Verification items for the finished model (mm, model axes). A direction names the side the tool comes from. Give positions to 0.01 mm unless a question says otherwise; leave off trailing zeros. Order: outer loops, then holes, each group sorted by start corner. A loop starts at its lowest first (then second) coordinate and runs counter-clockwise, first axis right, second up. Notation, with made-up numbers: (67.25, 17.25) - (99.25, 17.25) arc R27 ccw to (99.25, 46.25) - close; hole circle Ø2 at (2.25, 55). An arc over 180 degrees is marked (long way). Answer as a JSON object with one key per item and string values. Group by question number.
(1) Thickness scan on line 1 (Y direction, x = -239, z = 370); line 2 (Z direction, x = 136, y = -24). Record the ranges inside material, lowest first.
(2) Section check C-C (x = 239.5). Record the boundary of the cut face in (y, z), then the cut area to 3 significant figures.
(3) Mould release check, pull along Y, two halves, no side actions. Record for faces 4 (the face through (275.5, -4, 425)), 5 (the face through (-249, 223.3, 197)), 6 (the face through (-4, -275.5, 425)), 7 (the face through (-249, -223.3, 197)): +Y half, -Y half, draft (parallel to the pull), parting line (faces both ways), or undercut.
(4) Section check B-B (y = -133.5). Record the boundary of the cut face in (x, z).
(5) Depth check by flat-ended pin: pin 1 Ø13.5 at (y, z) = (240.5, 221) entering from -X; pin 2 Ø1 at (x, y) = (-216, 19.5) entering from -Z; pin 3 Ø23 at (y, z) = (-257, 281) entering from +X. Enter the tip coordinate at first touch or a pass-through.
(6) Access from +Z, -Z, +X, -X, +Y, -Y to the whole of each face (thin tool, end or side, straight path). Record for faces 1 (the face through (274, -249, 197)), 2 (the face through (-274, 248, 197)), 3 (the face through (248, -274, 197)).
(7) Section check A-A (z = 156). Count the separate pieces of the cut face and the enclosed holes in it, then the cut area to 3 significant figures.
```python
from build123d import *

# Parameters (mm, degrees)
F1_W     = 551
F1_H     = 551
F1_W_2   = 50.7
F1_H_2   = 50.7
F2_DEPTH = 50.1
F4_DEPTH = 400
F5_R     = 2.5
F6_R     = 1


with BuildPart() as f2:
    # F1 (on Top) → F2 (new body)
    with BuildSketch(Plane.XY):
        Rectangle(F1_W, F1_H)
        with Locations((-248.65, -248.65)):
            Rectangle(F1_W_2, F1_H_2, mode=Mode.SUBTRACT)
        with Locations((248.65, -248.65)):
            Rectangle(F1_W_2, F1_H_2, mode=Mode.SUBTRACT)
        with Locations((-248.65, 248.65)):
            Rectangle(F1_W_2, F1_H_2, mode=Mode.SUBTRACT)
        with Locations((248.65, 248.65)):
            Rectangle(F1_W_2, F1_H_2, mode=Mode.SUBTRACT)
        with Locations((-248.65, 248.65)):
            Rectangle(F1_W_2, F1_H_2)
        with Locations((248.65, 248.65)):
            Rectangle(F1_W_2, F1_H_2)
        with Locations((-248.65, -248.65)):
            Rectangle(F1_W_2, F1_H_2)
        with Locations((248.65, -248.65)):
            Rectangle(F1_W_2, F1_H_2)
    extrude(amount=-F2_DEPTH)


with BuildPart() as f2_1:
    # F3: moved
    add(f2.part.moved(Location((0, 0, 450))))

    # F1 (on Top) → F4 (join)
    with BuildSketch(Plane.XY):
        with Locations((-248.65, 248.65)):
            Rectangle(F1_W_2, F1_H_2)
        with Locations((248.65, -248.65)):
            Rectangle(F1_W_2, F1_H_2)
        with Locations((-248.65, -248.65)):
            Rectangle(F1_W_2, F1_H_2)
        with Locations((248.65, 248.65)):
            Rectangle(F1_W_2, F1_H_2)
    extrude(amount=F4_DEPTH)

    # F5
    f5_edges = [f2_1.edges().sort_by_distance(p)[0] for p in [
        (-274, -274, 199.95),
        (-274, 223.3, 199.95),
        (223.3, 223.3, 199.95),
        (223.3, -274, 199.95),
        (-223.3, -274, 199.95),
        (-223.3, 223.3, 199.95),
        (274, -274, 199.95),
        (274, 223.3, 199.95),
        (-223.3, -223.3, 199.95),
        (274, -223.3, 199.95),
        (-223.3, 274, 199.95),
        (274, 274, 199.95),
        (223.3, -223.3, 199.95),
        (-274, -223.3, 199.95),
        (223.3, 274, 199.95),
        (-274, 274, 199.95),
    ]]
    fillet(f5_edges, radius=F5_R)

    # F6
    f6_edges = [f2_1.edges().sort_by_distance(p)[0] for p in [
        (0, -275.5, 450),
        (275.5, 0, 450),
        (-275.5, 0, 450),
        (0, 275.5, 450),
        (275.5, -275.5, 424.95),
        (-275.5, -275.5, 424.95),
        (275.5, 275.5, 424.95),
        (-275.5, 275.5, 424.95),
    ]]
    fillet(f6_edges, radius=F6_R)


solid = f2_1.part
```
Solutions:
{
 "1": {"line 1": "y = -274 to -223.3, 223.3 to 274", "line 2": "z = 399.9 to 450"},
 "2": {"outline": "(-275.5, 399.9) - (-274, 399.9) - (-274, 0) - (-223.3, 0) - (-223.3, 399.9) - (223.3, 399.9) - (223.3, 0) - (274, 0) - (274, 399.9) - (275.5, 399.9) - (275.5, 449) arc R1 ccw to (274.5, 450) - (-274.5, 450) arc R1 ccw to (-275.5, 449) - close", "area": "68,200 mm2"},
 "3": {"face 4": "draft", "face 5": "undercut", "face 6": "-Y half", "face 7": "undercut"},
 "4": {"outline": "(-275.5, 399.9) - (275.5, 399.9) - (275.5, 449) arc R1 ccw to (274.5, 450) - (-274.5, 450) arc R1 ccw to (-275.5, 449) - close"},
 "5": {"pin 1": "stops at x = -274", "pin 2": "stops at z = 399.9", "pin 3": "stops at x = 274"},
 "6": {"face 1": "-Z, +X, +Y, -Y", "face 2": "-Z, -X, +Y, -Y", "face 3": "-Z, +X, -X, -Y"},
 "7": {"separate pieces": "4", "enclosed holes": "0", "area": "10,300 mm2"}
}
